```python
from build123d import *

# Parameters (mm, degrees)
ESQUISSE2_W             = 175
ESQUISSE2_H             = 3
BOSS_EXTRU_1_DEPTH      = 36.27
ESQUISSE3_R             = 2.5
ENL_V_MAT_EXTRU_1_DEPTH = 106.213182302
SKETCH1_W               = 175
SKETCH1_H               = 19.88750008
BOSS_EXTRUDE1_DEPTH     = 3


with BuildPart() as part:
    # Esquisse2 → Boss.-Extru.1 (new body)
    with BuildSketch(Plane(origin=(0, 0, 0), x_dir=(1, 0, 0), z_dir=(0, 1, 0))):
        with Locations((11.218290251, -2.666038947)):
            Rectangle(ESQUISSE2_W, ESQUISSE2_H)
    extrude(amount=BOSS_EXTRU_1_DEPTH)

    # Esquisse3 → Enlèv. mat.-Extru.1 (cut, through all)
    with BuildSketch(Plane.XY.offset(4.166038947)):
        with Locations((-53.031709749, 18.135)):
            Circle(ESQUISSE3_R)
        with Locations((75.468290251, 18.135)):
            Circle(ESQUISSE3_R)
    extrude(amount=-ENL_V_MAT_EXTRU_1_DEPTH, mode=Mode.SUBTRACT)

    # Sketch1 → Boss-Extrude1 (add)
    with BuildSketch(Plane.XY.offset(4.166038947)):
        with Locations((11.218290251, 46.21375004)):
            Rectangle(SKETCH1_W, SKETCH1_H)
    extrude(amount=-BOSS_EXTRUDE1_DEPTH)


solid = part.part
```
Could you check a few things on this model? Use its own coordinates, in mm. Coordinates: 2 decimals unless noted, no trailing zeros. Write each loop counter-clockwise with the first axis right and the second up, starting at its lowest first coordinate (ties: lowest second). Pieces come first, ordered by that corner, then holes. Notation, with made-up numbers: (-32, 20.25) -> (18, 20.25) arc R20 ccw to (18, 32.25) -> close; hole circle Ø11 at (37.25, -15.5). An arc over 180 degrees is marked (long way). One line per question, with ' | ' between items. Start each with the question number.
1. Please list where these lines run through material, in increasing order: line 1 along X through (y, z) = (20, 4.05); line 2 along X through (y, z) = (16, 2.85); line 3 along Y through (x, z) = (73.5, 2.1).
2. Will these pins go through, and if not, where does the flat tip stop? P1, Ø8, axis at x = -53.03, y = 18.14, coming from the -Z side; P2, Ø3, axis at x = 75.47, y = 18.14, coming from the +Z side.
3. If we section it at A-A (x = 74.5): Please give me the cut outline in (y, z), and give its area (3 significant figures).
4. Thinking about a two-plate mould opening in Y: for faces 1 (the face through (10, 56.158, 3)), 2 (the face through (77.85, 18.89, 2.69)), 3 (the face through (98.718, 28, 3)), which applies, pulls with the +Y half, pulls with the -Y half, needs draft (parallel to the pull), parting line crosses it, or undercut?
Return value:
1) line 1: x = -76.28 to -54.7, -51.37 to 73.8, 77.13 to 98.72 | line 2: x = -76.28 to -54.33, -51.73 to 74.17, 76.77 to 98.72 | line 3: y = 0 to 16.59, 19.68 to 56.16
2) P1: stops at z = 1.17 | P2: passes through
3) outline: (0, 1.17) -> (15.83, 1.17) -> (15.83, 4.17) -> (0, 4.17) -> close; (20.44, 1.17) -> (56.16, 1.17) -> (56.16, 4.17) -> (20.44, 4.17) -> close | area: 155 mm²
4) face 1: pulls with the +Y half | face 2: undercut | face 3: needs draft
